Geometry check sheet. Reference: the model listing, model coordinates, mm. Face numbers are marked on the shaded views. A direction names the side the tool comes from. Coordinates: 2 decimals unless noted, no trailing zeros. Loops run counter-clockwise (first coordinate to the right, second up) from the corner with the lowest first, then second, coordinate; pieces in that order, holes last. Notation, with made-up numbers: (82, 15.5) -> (120, 15.5) arc R21 ccw to (120, 20.5) -> close; hole circle Ø4 at (26, -11). An arc over 180 degrees is marked (long way). Answer as a JSON object with one key per item and string values.
from build123d import *

# Parameters (mm, degrees)
SKETCH1_W           = 54
SKETCH1_H           = 55
BOSS_EXTRUDE1_DEPTH = 30
SKETCH2_W           = 54
SKETCH2_H           = 15
CUT_EXTRUDE1_DEPTH  = 8
SKETCH3_R           = 2.5
CUT_EXTRUDE2_DEPTH  = 10
SKETCH4_R           = 2.5
CUT_EXTRUDE3_DEPTH  = 10


with BuildPart() as part:
    # Sketch1 → Boss-Extrude1 (new body)
    with BuildSketch(Plane.XY):
        with Locations((27, 27.5)):
            Rectangle(SKETCH1_W, SKETCH1_H)
    extrude(amount=BOSS_EXTRUDE1_DEPTH)

    # Sketch2 → Cut-Extrude1 (cut)
    with BuildSketch(Plane.XZ):
        with Locations((27, 15)):
            Rectangle(SKETCH2_W, SKETCH2_H)
    extrude(amount=-CUT_EXTRUDE1_DEPTH, mode=Mode.SUBTRACT)

    # Sketch3 → Cut-Extrude2 (cut)
    with BuildSketch(Plane(origin=(0, 55, 0), x_dir=(1, 0, 0), z_dir=(0, 1, 0))):
        with Locations(Location((19, -15, 0), (0, 0, 270))):
            Circle(SKETCH3_R)
        with Locations(Location((35, -15, 0), (0, 0, 270))):
            Circle(SKETCH3_R)
    extrude(amount=-CUT_EXTRUDE2_DEPTH, mode=Mode.SUBTRACT)

    # Sketch4 → Cut-Extrude3 (cut)
    with BuildSketch(Plane.XY.offset(30)):
        with Locations((27, 35.5)):
            Circle(SKETCH4_R)
        with Locations((27, 19.5)):
            Circle(SKETCH4_R)
    extrude(amount=-CUT_EXTRUDE3_DEPTH, mode=Mode.SUBTRACT)


solid = part.part
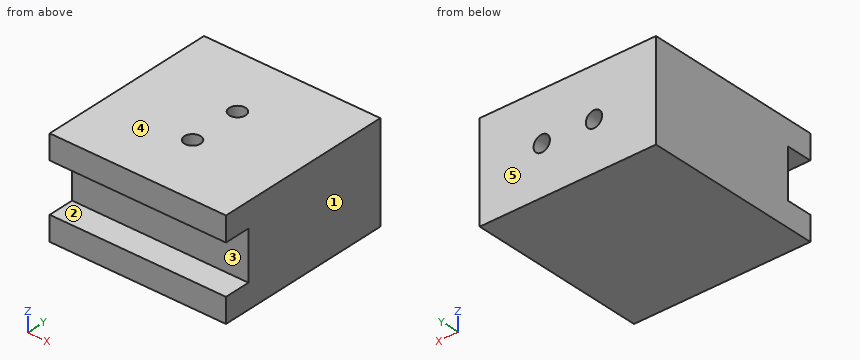
1. Thickness scan on probe 1 along X at (y, z) = (51, 15); probe 2 along Z at (x, y) = (46, 3); probe 3 along Y at (x, z) = (25.5, 28). Record the ranges inside material, lowest first. Write a range as from..to.
Evaluation:
{"probe 1": "x = 0..16.5, 21.5..32.5, 37.5..54", "probe 2": "z = 0..7.5, 22.5..30", "probe 3": "y = 0..17.5, 21.5..33.5, 37.5..55"}
2. Section check C-C, the plane z = 15. Record the boundary of the cut face in (x, y).
Evaluation:
{"outline": "(0, 8) -> (54, 8) -> (54, 55) -> (37.5, 55) -> (37.5, 45) -> (32.5, 45) -> (32.5, 55) -> (21.5, 55) -> (21.5, 45) -> (16.5, 45) -> (16.5, 55) -> (0, 55) -> close"}
3. Section check D-D, the plane y = 19.5. Record the boundary of the cut face in (x, z), then the cut area to 3 significant figures.
Evaluation:
{"outline": "(0, 0) -> (54, 0) -> (54, 30) -> (29.5, 30) -> (29.5, 20) -> (24.5, 20) -> (24.5, 30) -> (0, 30) -> close", "area": "1,570 mm^2"}
4. Tool access check on the marked faces 1 and 2. Record the directions out of +Z, -Z, +X, -X, +Y, -Y that give a thin tool (end or side, any length) a straight path to the whole face; none if there is none.
Evaluation:
{"face 1": "+Z, -Z, +X, +Y, -Y", "face 2": "+X, -X, -Y"}
5. Section check B-B, the plane x = 35. Record the boundary of the cut face in (y, z), then the cut area to 3 significant figures.
Evaluation:
{"outline": "(0, 0) -> (55, 0) -> (55, 12.5) -> (45, 12.5) -> (45, 17.5) -> (55, 17.5) -> (55, 30) -> (0, 30) -> (0, 22.5) -> (8, 22.5) -> (8, 7.5) -> (0, 7.5) -> close", "area": "1,480 mm^2"}
6. Section check A-A, the plane y = 7. Record the boundary of the cut face in (x, z), then the cut area to 3 significant figures.
Evaluation:
{"outline": "(0, 0) -> (54, 0) -> (54, 7.5) -> (0, 7.5) -> close; (0, 22.5) -> (54, 22.5) -> (54, 30) -> (0, 30) -> close", "area": "810 mm^2"}
7. Mould release check, pull along Y, two halves, no side actions. Record for the marked faces 3, 4 and 5: released by +Y, released by -Y, zero draft, split by the parting line, or undercut.
Evaluation:
{"face 3": "released by -Y", "face 4": "zero draft", "face 5": "released by +Y"}
8. Depth check by flat-ended pin: P1, Ø6, axis at x = 36.5, z = 20.5, coming from the -Y side; P2, Ø1.5, axis at x = 28, y = 34.5, coming from the +Z side; P3, Ø3, axis at x = 35, z = 15, coming from the -Y side; P4, Ø1.5, axis at x = 18.5, z = 15.5, coming from the +Y side. Enter the tip coordinate at first touch or a pass-through.
Evaluation:
{"P1": "stops at y = 0", "P2": "stops at z = 20", "P3": "stops at y = 8", "P4": "stops at y = 45"}
